from build123d import *

# Parameters (mm, degrees)
SKETCH1_W                                       = 30
SKETCH1_H                                       = 10
BOSS_EXTRUDE1_DEPTH                             = 7.5
CSK_FOR_M3_FLAT_HEAD_MACHINE_SCREW1_D           = 3.2
CSK_FOR_M3_FLAT_HEAD_MACHINE_SCREW1_CSINK_D     = 6.3
CSK_FOR_M3_FLAT_HEAD_MACHINE_SCREW1_CSINK_ANGLE = 90
M5_CLEARANCE_HOLE1_D                            = 5.3
FILLET1_R                                       = 0.5


with BuildPart() as part:
    # Sketch1 → Boss-Extrude1 (new body)
    with BuildSketch(Plane(origin=(0, 0, 0), x_dir=(1, 0, 0), z_dir=(0, 1, 0))):
        Rectangle(SKETCH1_W, SKETCH1_H)
    extrude(amount=-BOSS_EXTRUDE1_DEPTH)

    # CSK for M3 Flat Head Machine Screw1 (through all)
    with Locations(Plane(origin=(-10, 0, 0), x_dir=(0, 0, 1), z_dir=(0, 1, 0))):
        with Locations((0, 0), (0, 20)):
            CounterSinkHole(CSK_FOR_M3_FLAT_HEAD_MACHINE_SCREW1_D / 2, CSK_FOR_M3_FLAT_HEAD_MACHINE_SCREW1_CSINK_D / 2, counter_sink_angle=CSK_FOR_M3_FLAT_HEAD_MACHINE_SCREW1_CSINK_ANGLE)

    # M5 Clearance Hole1 (through all)
    with Locations(Plane.ZX):
        with Locations((0, 0)):
            Hole(M5_CLEARANCE_HOLE1_D / 2)

    # Fillet1
    fillet1_edges = [part.edges().sort_by_distance(p)[0] for p in [
        (-15, -3.75, -5),
        (15, -3.75, -5),
        (15, -3.75, 5),
        (-15, -3.75, 5),
    ]]
    fillet(fillet1_edges, radius=FILLET1_R)


solid = part.part
Here's how the part is built. I have some questions about the finished solid (model axes, mm). Coordinates: 2 decimals unless noted, no trailing zeros. Write each loop counter-clockwise with the first axis right and the second up, starting at its lowest first coordinate (ties: lowest second). Pieces come first, ordered by that corner, then holes.
Item 1: If we mould it in two halves opening along Z, with no side actions, what happens to faces 1 (the flat face through (15, -4, 0)), 2 (the flat face through (0, -4, -5)), 3 (the flat face through (0, -4, 5)), 4 (the cylindrical face through (-1.01, -3.8, -2.45))? For each: +Z half, -Z half, draft (parallel to the pull), parting line (faces both ways), or undercut.
Item 2: If I drill on line 1 (X direction, y = -3.65, z = 0); line 2 (X direction, y = -3, z = -0.5); line 3 (Z direction, x = -10, y = -3.3), over which ranges is the centre line in solid material (lowest first)?
Item 3: I want a section at C-C on y = -1. Write out the boundary of the cut face in (x, z).
Item 4: I want a section at A-A on x = 10. Write out the boundary of the cut face in (y, z).
Item 5: I want a section at D-D on y = -4. Write out the boundary of the cut face in (x, z), and give its area (3 significant figures).
Item 6: I want a section at B-B on z = 0. Write out the boundary of the cut face in (x, y), and give its area (3 significant figures).
Findings below:
1. face 1: draft
1. face 2: -Z half
1. face 3: +Z half
1. face 4: undercut
2. line 1: x = -15 to -11.6, -8.4 to -2.65, 2.65 to 8.4, 11.6 to 15
2. line 2: x = -15 to -11.52, -8.48 to -2.6, 2.6 to 8.48, 11.52 to 15
2. line 3: z = -5 to -1.6, 1.6 to 5
3. outline: (-15, -4.5) arc R0.5 ccw to (-14.5, -5) - (14.5, -5) arc R0.5 ccw to (15, -4.5) - (15, 4.5) arc R0.5 ccw to (14.5, 5) - (-14.5, 5) arc R0.5 ccw to (-15, 4.5) - close; hole circle Ø4.3 at (-10, 0); hole circle Ø5.3 at (0, 0); hole circle Ø4.3 at (10, 0)
4. outline: (-7.5, -5) - (0, -5) - (0, -3.15) - (-1.55, -1.6) - (-7.5, -1.6) - close; (-7.5, 1.6) - (-1.55, 1.6) - (0, 3.15) - (0, 5) - (-7.5, 5) - close
5. outline: (-15, -4.5) arc R0.5 ccw to (-14.5, -5) - (14.5, -5) arc R0.5 ccw to (15, -4.5) - (15, 4.5) arc R0.5 ccw to (14.5, 5) - (-14.5, 5) arc R0.5 ccw to (-15, 4.5) - close; hole circle Ø3.2 at (-10, 0); hole circle Ø5.3 at (0, 0); hole circle Ø3.2 at (10, 0)
5. area: 262 mm2
6. outline: (-15, -7.5) - (-11.6, -7.5) - (-11.6, -1.55) - (-13.15, 0) - (-15, 0) - close; (-8.4, -7.5) - (-2.65, -7.5) - (-2.65, 0) - (-6.85, 0) - (-8.4, -1.55) - close; (2.65, -7.5) - (8.4, -7.5) - (8.4, -1.55) - (6.85, 0) - (2.65, 0) - close; (11.6, -7.5) - (15, -7.5) - (15, 0) - (13.15, 0) - (11.6, -1.55) - close
6. area: 132 mm2
